from build123d import *

# Parameters (mm, degrees)
F1_DEPTH       = 25
F3_D           = 5.2
F3_CBORE_D     = 10
F3_CBORE_DEPTH = 5.2
F4_D           = 6
F5_SIZE        = 1


with BuildPart() as f1:
    # F0 (on Right) → F1 (new body, symmetric)
    with BuildSketch(Plane.YZ):
        Polygon((10, 4.5), (-10, 4.5), (-10, -4.5), (-2.5, -4.5), (-2.5, -7.5), (2.5, -7.5), (2.5, -4.5), (10, -4.5), align=None)
    extrude(amount=F1_DEPTH, both=True)

    # F3 (through all)
    with Locations(Plane.XY.offset(4.5)):
        with Locations((-15, 0), (15, 0)):
            CounterBoreHole(F3_D / 2, F3_CBORE_D / 2, F3_CBORE_DEPTH)

    # F4 (through all)
    with Locations(Plane.XY.offset(4.5)):
        with Locations((0, 0)):
            Hole(F4_D / 2)

    # F5
    f5_edges = [f1.edges().sort_by_distance(p)[0] for p in [
        (25, -10, 0),
        (25, 10, 0),
        (-25, -10, 0),
        (-25, 10, 0),
    ]]
    chamfer(f5_edges, length=F5_SIZE)


solid = f1.part
Input: part model. Units: mm. Frame: model coordinates. A direction names the side the tool comes from. Give positions to 0.01 mm unless a question says otherwise; leave off trailing zeros. Loops run counter-clockwise (first coordinate to the right, second up) from the corner with the lowest first, then second, coordinate; pieces in that order, holes last. Notation, with made-up numbers: (40, 53.25) - (99, 53.25) arc R32 cw to (99, 91.25) - close; hole circle Ø7 at (8, -19.5). An arc over 180 degrees is marked (long way). Use CSV: the item, a comma, the result in double quotes. Start each with the question number.
Item 1: Section B-B on z = -6.25. Return loops of the section in (x, y).
Item 2: Reachability of faces 1 (the flat face through (-24.5, 9.5, -0.1)), 2 (the flat face through (8, 2.5, -6)), 3 (the flat face through (-8, -2.5, -6)) from +Z, -Z, +X, -X, +Y, -Y: full face, straight path, thin tool, end or side. Return the list, or none.
Item 3: Contact query for flat-ended pins moving along their axis: P1, Ø0.9, axis at x = -21.5, z = -6.5, coming from the +Y side; P2, Ø3, axis at x = 13.5, y = -2.5, coming from the +Z side; P3, Ø3, axis at x = -5, y = 6, coming from the -Z side. Output: stop coordinate, or through.
Item 4: Section C-C on z = 2.25. Return loops of the section in (x, y).
Item 5: Section D-D on y = 1. Return loops of the section in (x, z), then the cut area to 3 significant figures.
Item 6: Line query: line 1 (X direction, y = 0, z = -5.5); line 2 (Y direction, x = -15, z = 0.8); line 3 (Y direction, x = -15, z = -3.25). Output: solid intervals per line, ascending.
Item 7: Mould query, pull axis Y, two halves, no side actions, for faces 4 (the flat face through (20, 2.5, -6)), 5 (the flat face through (25, 0, 0)), 6 (the flat face through (-13, -2, -0.7)). Classes: pulls with the +Y half, pulls with the -Y half, needs draft (parallel to the pull), parting line crosses it, or undercut.
Item 8: Section A-A on x = 0. Return loops of the section in (y, z).
Ans:
1,outline,"(-25, -2.5) - (-15.71, -2.5) arc R2.6 cw to (-15.71, 2.5) - (-25, 2.5) - close; (-14.29, -2.5) - (-1.66, -2.5) arc R3 cw to (-1.66, 2.5) - (-14.29, 2.5) arc R2.6 cw to start; (1.66, -2.5) - (14.29, -2.5) arc R2.6 cw to (14.29, 2.5) - (1.66, 2.5) arc R3 cw to start; (15.71, -2.5) - (25, -2.5) - (25, 2.5) - (15.71, 2.5) arc R2.6 cw to start"
2,face 1,"+Z, -Z, -X, +Y"
2,face 2,"-Z, +X, -X, +Y"
2,face 3,"-Z, +X, -X, -Y"
3,P1,"stops at y = 2.5"
3,P2,"stops at z = -0.7"
3,P3,"stops at z = -4.5"
4,outline,"(-25, -9) - (-24, -10) - (24, -10) - (25, -9) - (25, 9) - (24, 10) - (-24, 10) - (-25, 9) - close; hole circle Ø10 at (-15, 0); hole circle Ø6 at (0, 0); hole circle Ø10 at (15, 0)"
5,outline,"(-25, -7.5) - (-17.4, -7.5) - (-17.4, -0.7) - (-19.9, -0.7) - (-19.9, 4.5) - (-25, 4.5) - close; (-12.6, -7.5) - (-2.83, -7.5) - (-2.83, 4.5) - (-10.1, 4.5) - (-10.1, -0.7) - (-12.6, -0.7) - close; (2.83, -7.5) - (12.6, -7.5) - (12.6, -0.7) - (10.1, -0.7) - (10.1, 4.5) - (2.83, 4.5) - close; (17.4, -7.5) - (25, -7.5) - (25, 4.5) - (19.9, 4.5) - (19.9, -0.7) - (17.4, -0.7) - close"
5,area,"365 mm2"
6,line 1,"x = -25 to -17.6, -12.4 to -3, 3 to 12.4, 17.6 to 25"
6,line 2,"y = -10 to -5, 5 to 10"
6,line 3,"y = -10 to -2.6, 2.6 to 10"
7,face 4,"pulls with the +Y half"
7,face 5,"needs draft"
7,face 6,"undercut"
8,outline,"(-10, -4.5) - (-3, -4.5) - (-3, 4.5) - (-10, 4.5) - close; (3, -4.5) - (10, -4.5) - (10, 4.5) - (3, 4.5) - close"
